For this review, take the finished solid that the model builds, in its own axes (mm). A direction names the side the tool comes from. Round coordinates to 2 decimals unless told otherwise and drop trailing zeros. Order: outer loops, then holes, each group sorted by start corner. A loop starts at its lowest first (then second) coordinate and runs counter-clockwise, first axis right, second up. Notation, with made-up numbers: M 41,0.5 L 75,0.5 A30 cw 75,27.5 Z; hole C -14.75,83 d3. An arc over 180 degrees is marked long. Write item = value, one per line. Start each with the question number.
from build123d import *

# Parameters (mm, degrees)
SKETCH1_R           = 35
BOSS_EXTRUDE1_DEPTH = 10
SKETCH2_R           = 20.280215245
SKETCH2_R_2         = 15.321162536
CUT_EXTRUDE1_DEPTH  = 2
SKETCH3_R           = 4
BOSS_EXTRUDE2_DEPTH = 25.4


with BuildPart() as part:
    # Sketch1 → Boss-Extrude1 (new body)
    with BuildSketch(Plane(origin=(0, 0, 0), x_dir=(1, 0, 0), z_dir=(0, 1, 0))):
        Circle(SKETCH1_R)
    extrude(amount=BOSS_EXTRUDE1_DEPTH)

    # Sketch2 → Cut-Extrude1 (cut)
    with BuildSketch(Plane(origin=(0, 10, 0), x_dir=(1, 0, 0), z_dir=(0, 1, 0))):
        Circle(SKETCH2_R)
        Circle(SKETCH2_R_2, mode=Mode.SUBTRACT)
    extrude(amount=-CUT_EXTRUDE1_DEPTH, mode=Mode.SUBTRACT)

    # Sketch3 → Boss-Extrude2 (add)
    with BuildSketch(Plane.XZ):
        Circle(SKETCH3_R)
    extrude(amount=BOSS_EXTRUDE2_DEPTH)


solid = part.part
(1) We need section B-B, the plane x = 0. Write out the cut boundary in (y, z), then the cut area to 3 significant figures.
(2) For faces 4 (the cylindrical face through (-4.396, 9.014, 19.798)), 5 (the flat face through (15, 10, 15)), list the 3-axis set-ups (+Z, -Z, +X, -X, +Y, -Y) from which the entire face can be reached by the end or side of a thin tool; tool diameter is ignored.
(3) We need section D-D, the plane z = 17.5. Write out the cut boundary in (x, y).
(4) Insertion check: pin 1 (2 mm diameter, centred on y = 4, z = 27, fed in from -X); pin 2 (5 mm diameter, centred on y = 0.5, z = -26.5, fed in from -X); pin 3 (10 mm diameter, centred on x = 8.5, z = 16.5, fed in from -Y). Each pin has a flat end and moves straight along its axis. Give the tip position at first contact, or say it passes through.
(5) Draft analysis for pull direction X (two halves, no side actions). For faces 1 (the flat face through (0, 10, 0)), 2 (the flat face through (7, 8, -14)), 3 (the cylindrical face through (-0.867, -12.522, -3.905)), state which applies: released by +X, released by -X, zero draft, split by the parting line, or undercut.
(6) We need section A-A, the plane z = 0. Write out the cut boundary in (x, y), then the cut area to 3 significant figures.
(7) For line 1 along X through (y, z) = (9, 0); line 2 along Y through (x, z) = (27.5, 9.5), list the stretches that pass through material, from the lowest coordinate up.
(8) We need section C-C, the plane y = 2.5. Write out the cut boundary in (x, z), then the cut area to 3 significant figures.
Values:
q1.outline = M -25.4,-4 L 0,-4 L 0,-35 L 10,-35 L 10,-20.28 L 8,-20.28 L 8,-15.32 L 10,-15.32 L 10,15.32 L 8,15.32 L 8,20.28 L 10,20.28 L 10,35 L 0,35 L 0,4 L -25.4,4 Z
q1.area = 883 mm²
q2.face_4 = +Y
q2.face_5 = +Z, -Z, +X, -X, +Y
q3.outline = M -30.31,0 L 30.31,0 L 30.31,10 L 10.25,10 L 10.25,8 L -10.25,8 L -10.25,10 L -30.31,10 Z
q4.pin_1 = -23.43
q4.pin_2 = -25.48
q4.pin_3 = 0
q5.face_1 = zero draft
q5.face_2 = undercut
q5.face_3 = split by the parting line
q6.outline = M -35,0 L -4,0 L -4,-25.4 L 4,-25.4 L 4,0 L 35,0 L 35,10 L 20.28,10 L 20.28,8 L 15.32,8 L 15.32,10 L -15.32,10 L -15.32,8 L -20.28,8 L -20.28,10 L -35,10 Z
q6.area = 883 mm²
q7.line_1 = -35 to -20.28, -15.32 to 15.32, 20.28 to 35
q7.line_2 = 0 to 10
q8.outline = C 0,0 d70
q8.area = 3,850 mm²
